from build123d import *

# Parameters (mm, degrees)
SKETCH1_R           = 20.32
BOSS_EXTRUDE1_DEPTH = 58.70448
SHELL1_T            = -2.54
SKETCH2_R           = 3.96875
CUT_EXTRUDE1_DEPTH  = 64.089251174
CIRPATTERN1_COUNT   = 3
SKETCH9_R           = 20.32
CUT_EXTRUDE2_DEPTH  = 4.318


with BuildPart() as part:
    # Sketch1 → Boss-Extrude1 (new body)
    with BuildSketch(Plane(origin=(0, 0, 0), x_dir=(1, 0, 0), z_dir=(0, 1, 0))):
        with Locations(Location((0, 0, 0), (0, 0, 270))):
            Circle(SKETCH1_R)
    extrude(amount=BOSS_EXTRUDE1_DEPTH)

    # Shell1
    shell1_openings = [part.faces().sort_by_distance(p)[0] for p in [
        (0, 0, 0),
    ]]
    offset(amount=SHELL1_T, openings=shell1_openings, kind=Kind.INTERSECTION)

    # Sketch2 → Cut-Extrude1 (cut, through all)
    with BuildSketch(Plane.XZ.offset(-56.16448)):
        with Locations(Location((0, 0, 0), (0, 0, 270))):
            Circle(SKETCH2_R)
    extrude(amount=-CUT_EXTRUDE1_DEPTH, mode=Mode.SUBTRACT)

    # Sketch8 → #2 Clearance Hole1 (revolve, cut)
    with BuildSketch(Plane(origin=(-2.56879902, 7.424974445, 20.156975755), x_dir=(0.9919771533037619, 0, 0.1264172746240199), z_dir=(0, 1, 0))):
        Polygon((0, 0), (0, 9.838434313), (1.1303, 8.89), (1.1303, 0), align=None)
    f_2_clearance_hole1 = revolve(axis=Axis((-3.371548714, 7.424974445, 26.456030679), (0.1264172746240199, 0, -0.9919771533037619)), mode=Mode.SUBTRACT)

    # CirPattern1: #2 Clearance Hole1 ×3 about axis
    cirpattern1_axis = Axis((0, 58.70448, 0), (0, -1, 0))
    for i in range(1, CIRPATTERN1_COUNT):
        add(f_2_clearance_hole1.rotate(cirpattern1_axis, i * 360 / CIRPATTERN1_COUNT), mode=Mode.SUBTRACT)

    # Sketch9 → Cut-Extrude2 (cut)
    with BuildSketch(Plane.XZ):
        with Locations(Location((0, 0, 0), (0, 0, 270))):
            Circle(SKETCH9_R)
    extrude(amount=-CUT_EXTRUDE2_DEPTH, mode=Mode.SUBTRACT)


solid = part.part
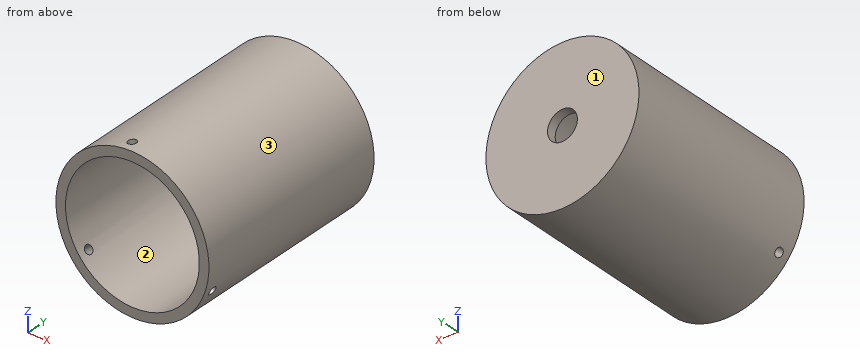
Input: part model. Units: mm. Frame: model coordinates. Face numbers are marked on the shaded views. Coordinates: 2 decimals unless noted, no trailing zeros. Write each loop counter-clockwise with the first axis right and the second up, starting at its lowest first coordinate (ties: lowest second). Pieces come first, ordered by that corner, then holes. Notation, with made-up numbers: M -10,-11.5 L 28,-11.5 A20 cw 28,23.5 Z; hole C 74.25,66.25 d5. An arc over 180 degrees is marked long. Answer as a JSON object with one key per item and string values. Group by question number.
(1) Section C-C on x = -6. Output: boundary loops of the cut face in (y, z), plus the area to 3 significant figures.
(2) Mould query, pull axis X, two halves, no side actions, for the marked faces 1, 2 and 3. Classes: pulls with the +X half, pulls with the -X half, needs draft (parallel to the pull), parting line crosses it, or undercut.
(3) Section B-B on z = 0. Output: boundary loops of the cut face in (x, y).
(4) Contact query for flat-ended pins moving along their axis: P1, Ø1, axis at y = 15.5, z = 12, coming from the -X side; P2, Ø10, axis at x = -0.5, y = 12.5, coming from the -Z side; P3, Ø10.5, axis at x = -1, z = -6.5, coming from the -Y side; P4, Ø5, axis at y = 39, z = -13.5, coming from the -X side. Output: stop coordinate, or through.
(5) Section A-A on x = 0. Output: boundary loops of the cut face in (y, z).
(6) Section D-D on y = 52. Output: boundary loops of the cut face in (x, z), plus the area to 3 significant figures.
(7) Ray query, line 1 along X through (y, z) = (41.5, 0); line 2 along X through (y, z) = (56.75, 0); line 3 along Y through (x, z) = (12, 0.5). Return the intervals inside material, ascending. Write a range as [from, to].
Result set:
{
 "1": {"outline": "M 4.32,-19.41 L 58.7,-19.41 L 58.7,19.41 L 4.32,19.41 L 4.32,16.74 L 56.16,16.74 L 56.16,-16.74 L 4.32,-16.74 Z", "area": "376 mm2"},
 "2": {"face 1": "needs draft", "face 2": "undercut", "face 3": "parting line crosses it"},
 "3": {"outline": "M -20.32,4.32 L -17.78,4.32 L -17.78,56.16 L -3.97,56.16 L -3.97,58.7 L -20.32,58.7 Z; M 3.97,56.16 L 17.78,56.16 L 17.78,4.32 L 20.32,4.32 L 20.32,58.7 L 3.97,58.7 Z"},
 "4": {"P1": "stops at x = -16.75", "P2": "stops at z = -20.32", "P3": "stops at y = 56.16", "P4": "stops at x = -17.09"},
 "5": {"outline": "M 4.32,-20.32 L 58.7,-20.32 L 58.7,-3.97 L 56.16,-3.97 L 56.16,-17.78 L 4.32,-17.78 Z; M 4.32,17.78 L 56.16,17.78 L 56.16,3.97 L 58.7,3.97 L 58.7,20.32 L 4.32,20.32 Z"},
 "6": {"outline": "C 0,0 d40.64; hole C 0,0 d35.56", "area": "304 mm2"},
 "7": {"line 1": "x = [-20.32, -17.78], [17.78, 20.32]", "line 2": "x = [-20.32, -3.97], [3.97, 20.32]", "line 3": "y = [56.16, 58.7]"}
}
